CAD build for the part. Positions are in the model's coordinates, mm. A direction names the side the tool comes from. Round coordinates to 2 decimals unless told otherwise and drop trailing zeros. One line per question, with ' | ' between items.
```python
from build123d import *

# Parameters (mm, degrees)
F0_W           = 200.025
F0_H           = 76.2
F1_DEPTH       = 25.4
F3_D           = 3.4
F3_CBORE_D     = 6.5
F3_CBORE_DEPTH = 3


with BuildPart() as f1:
    # F0 (on Top) → F1 (new body)
    with BuildSketch(Plane.XY):
        with Locations((100.0125, 38.1)):
            Rectangle(F0_W, F0_H)
    extrude(amount=F1_DEPTH)

    # F3 (through all)
    with Locations(Plane.XY.offset(25.4)):
        with Locations((4.9625, 60.2), (29.9625, 60.2), (4.9625, 16), (29.9625, 16), (170.0625, 60.2), (195.0625, 60.2), (170.0625, 16), (195.0625, 16)):
            CounterBoreHole(F3_D / 2, F3_CBORE_D / 2, F3_CBORE_DEPTH)


solid = f1.part
```
(1) Tool access for faces 3 (the face through (196.5, 58.8, 22.4)), 4 (the face through (30.33, 58.54, 11.04)): list every direction of +Z, -Z, +X, -X, +Y, -Y with a clear straight run to the whole face (end or side of a thin tool).
Results found:
face 3: +Z | face 4: +Z, -Z
(2) Two-plate mould, pull along Y, no slides. Class faces 1 (the face through (6.4, 58.8, 22.4)), 2 (the face through (99, 39, 0)): released by +Y, released by -Y, zero draft, split by the parting line, or undercut.
Results found:
face 1: undercut | face 2: zero draft
(3) Drop a flat-ended pin along its axis: P1, Ø4, axis at x = 29.96, y = 16, coming from the +Z side. Give the stop position or say it passes through.
Results found:
P1: stops at z = 22.4
(4) Probe L1, parallel to Y at x = 30.5, z = 19; L2, parallel to Y at x = 28, z = 24; L3, parallel to X at y = 15.5, z = 22.25 (3 decimals). List the from-to ranges inside material, lowest first.
Results found:
L1: y = 0 to 14.39, 17.61 to 58.59, 61.81 to 76.2 | L2: y = 0 to 13.41, 18.59 to 57.61, 62.79 to 76.2 | L3: x = 0 to 3.338, 6.587 to 28.338, 31.587 to 168.438, 171.687 to 193.438, 196.687 to 200.025
